Can you work these out from the model? Positions are in its coordinate system, mm. A direction names the side the tool comes from. Round coordinates to 2 decimals unless told otherwise and drop trailing zeros. Loops run counter-clockwise (first coordinate to the right, second up) from the corner with the lowest first, then second, coordinate; pieces in that order, holes last. Notation, with made-up numbers: (69, 80) -> (79, 80) arc R19 ccw to (79, 104) -> close; hole circle Ø5 at (45, 2). An arc over 180 degrees is marked (long way). Answer as a JSON object with one key per item and string values.
```python
from build123d import *

# Parameters (mm, degrees)
SKETCH014_W      = 2.5
SKETCH014_H      = 3.5
EXTRUDE015_DEPTH = 4.5
EXTRUDE014_DEPTH = 6.6
SKETCH039_R      = 1.5
EXTRUDE047_DEPTH = 0.5


with BuildPart() as extrude015:
    # Sketch014 → Extrude015 (new body)
    with BuildSketch(Plane(origin=(0, 0, -10), x_dir=(1, 0, 0), z_dir=(0, 0, -1))):
        Rectangle(SKETCH014_W, SKETCH014_H)
    extrude(amount=-EXTRUDE015_DEPTH)


with BuildPart() as extrude015_1:
    # Extrude015 placement: moved
    add(extrude015.part.moved(Location((0, 0, 10))))


with BuildPart() as cap003:
    # Sketch013 → Extrude014 (new body)
    with BuildSketch(Plane.XZ.offset(10)):
        Polygon((-3.3, 7), (3.3, 7), (3.3, 1), (4.3, 1), (4.3, 0), (-4.3, 0), (-4.3, 1), (-3.3, 1), align=None)
    extrude(amount=-EXTRUDE014_DEPTH)


with BuildPart() as cap003_1:
    # Extrude014 placement: moved
    add(cap003.part.moved(Location((0, 6.75, 0))))

    # Cut023: cut Extrude015
    add(extrude015_1.part, mode=Mode.SUBTRACT)


with BuildPart() as shutter:
    # Sketch039 → Extrude047 (new body)
    with BuildSketch(Plane.XY.offset(20)):
        Circle(SKETCH039_R)
    extrude(amount=EXTRUDE047_DEPTH)


with BuildPart() as shutter_1:
    # Extrude047 placement: moved
    add(shutter.part.moved(Location((0, 0, -13))))

    # Fusion035: union cap003
    add(cap003_1.part)


with BuildPart() as shutter_2:
    # Fusion035 placement: moved
    add(shutter_1.part.moved(Location((-22.5, 0, 50))))


solid = shutter_2.part
```
Q1. I'm going to push flat-ended pins straight in: pin 1 (1.1 mm diameter, centred on x = -18.5, y = -0.5, fed in from +Z); pin 2 (0.8 mm diameter, centred on x = -22, y = -0.5, fed in from -Z); pin 3 (1.8 mm diameter, centred on y = -1, z = 53.5, fed in from -X). Where does each tip first touch, or does it pass through?
Determined:
{"pin 1": "z = 51", "pin 2": "z = 54.5", "pin 3": "x = -25.8"}
Q2. I want a section at B-B, the plane x = -22.5. Write out the boundary of the cut face in (y, z), then the cut area to 4 significant figures.
Determined:
{"outline": "(-3.25, 50) -> (-1.75, 50) -> (-1.75, 54.5) -> (1.75, 54.5) -> (1.75, 50) -> (3.35, 50) -> (3.35, 57) -> (1.5, 57) -> (1.5, 57.5) -> (-1.5, 57.5) -> (-1.5, 57) -> (-3.25, 57) -> close", "area": "31.95 mm²"}
Q3. I want a section at D-D, the plane y = 2. Write out the boundary of the cut face in (x, z), then the cut area to 3 significant figures.
Determined:
{"outline": "(-26.8, 50) -> (-18.2, 50) -> (-18.2, 51) -> (-19.2, 51) -> (-19.2, 57) -> (-25.8, 57) -> (-25.8, 51) -> (-26.8, 51) -> close", "area": "48.2 mm²"}
Q4. If I drill on L1, parallel to X at y = 0.75, z = 51.25; L2, parallel to X at y = 1.5, z = 50.75; L3, parallel to Y at x = -22.75, z = 51.75, over which ranges is the centre line in solid material (lowest first)? Write a range as [from, to].
Determined:
{"L1": "[-25.8, -23.75], [-21.25, -19.2]", "L2": "[-26.8, -23.75], [-21.25, -18.2]", "L3": "[-3.25, -1.75], [1.75, 3.35]"}
Q5. On a 3-axis mill with a long thin cutter (end or side, diameter ignored), from which of +Z, -Z, +X, -X, +Y, -Y can I reach the whole of each face in a straight line? I mean faces 4 (the flat face through (-19.2, 0, 54)), 5 (the flat face through (-25.8, 0, 54)), 6 (the cylindrical face through (-24, 0.07, 57.25)), 7 (the flat face through (-22, -3.25, 54)), 8 (the flat face through (-23, 0, 54.5)). Say none if no direction works.
Determined:
{"face 4": "+Z, +X, +Y, -Y", "face 5": "+Z, -X, +Y, -Y", "face 6": "+Z", "face 7": "+Z, -Z, +X, -X, -Y", "face 8": "-Z"}
Q6. I want a section at A-A, the plane z = 53.75. Write out the boundary of the cut face in (x, y).
Determined:
{"outline": "(-25.8, -3.25) -> (-19.2, -3.25) -> (-19.2, 3.35) -> (-25.8, 3.35) -> close; hole (-23.75, -1.75) -> (-21.25, -1.75) -> (-21.25, 1.75) -> (-23.75, 1.75) -> close"}
Q7. I want a section at C-C, the plane y = 0. Write out the boundary of the cut face in (x, z).
Determined:
{"outline": "(-26.8, 50) -> (-23.75, 50) -> (-23.75, 54.5) -> (-21.25, 54.5) -> (-21.25, 50) -> (-18.2, 50) -> (-18.2, 51) -> (-19.2, 51) -> (-19.2, 57) -> (-21, 57) -> (-21, 57.5) -> (-24, 57.5) -> (-24, 57) -> (-25.8, 57) -> (-25.8, 51) -> (-26.8, 51) -> close"}
Q8. We'd pull the mould along Y, two halves only. Please class faces 1 (the flat face through (-19, 0, 51)), 2 (the flat face through (-22, 3.35, 54)), 3 (the flat face through (-23, -1.75, 52)): pulls with the +Y half, pulls with the -Y half, needs draft (parallel to the pull), parting line crosses it, or undercut.
Determined:
{"face 1": "needs draft", "face 2": "pulls with the +Y half", "face 3": "undercut"}
